Input: part model. Units: mm. Frame: model coordinates. A direction names the side the tool comes from. Coordinates: 2 decimals unless noted, no trailing zeros. Loops run counter-clockwise (first coordinate to the right, second up) from the corner with the lowest first, then second, coordinate; pieces in that order, holes last. Notation, with made-up numbers: (79.5, -3.5) -> (105.5, -3.5) arc R21 cw to (105.5, 32.5) -> close; hole circle Ø7 at (61, -17). An arc over 180 degrees is marked (long way). Put each result on its own line as item: value. Start each with the question number.
1) Set-up query: faces 1 (the flat face through (-1.5, 9, 30)), 2 (the flat face through (-33, 1.5, 8)), 3 (the flat face through (1.574, 31.563, 7.814)). Return all of +Z, -Z, +X, -X, +Y, -Y with unobstructed straight access to the full face (end or side cutting, diameter ignored); none if empty.
2) Cut plane C-C (x = -12.5). Return the cut outline in (y, z), plus the area to 3 significant figures.
3) Cut plane A-A (z = 6). Return the cut outline in (x, y), plus the area to 3 significant figures.
4) Contact query for flat-ended pins moving along their axis: P1, Ø2, axis at x = -27.5, z = 14.5, coming from the -Y side; P2, Ø8, axis at x = -32.5, y = 11, coming from the +Z side; P3, Ø2, axis at x = -19, z = 24.5, coming from the +Y side; P4, Ø13, axis at y = 11, z = 26.5, coming from the +X side. Output: stop coordinate, or through.
5) Cut plane D-D (x = -25.5). Return the cut outline in (y, z), plus the area to 3 significant figures.
6) Material intervals for L1, parallel to X at y = 15.5, z = 2; L2, parallel to Z at x = -7.5, y = 44; L3, parallel to Y at x = -3.5, z = 36, sorted ascending.
7) Cut plane B-B (y = 16). Return the cut outline in (x, z), plus the area to 3 significant figures.
from build123d import *

# Parameters (mm, degrees)
F1_DEPTH = 15.85
F3_DEPTH = 1.6
F4_W     = 16.05
F4_H     = 16.05
F5_DEPTH = 25.4


with BuildPart() as f1:
    # F0 (on Top) → F1 (new body)
    with BuildSketch(Plane.XY):
        Polygon((-19.63319, 0), (0, 0), (0, 19.05), (-1.455444, 19.412883), (4.689373, 44.058394), (-10.883874, 47.941241), (-17.02869, 23.295729), (-18.484134, 23.658612), (-19.63319, 19.05), (-19.63319, 17.55), (-45.03319, 17.55), (-45.03319, 1.5), (-19.63319, 1.5), align=None)
    extrude(amount=F1_DEPTH)

    # F2 (on face) → F3 (join)
    with BuildSketch(Plane.XY.offset(15.85)):
        Polygon((-19.63319, 1.5), (-19.63319, 0), (0, 0), (0, 19.05), (-1.455444, 19.412883), (-17.02869, 23.295729), (-18.484134, 23.658612), (-19.63319, 19.05), (-19.63319, 17.55), align=None)
    extrude(amount=F3_DEPTH)

    # F4 (on face) → F5 (join)
    with BuildSketch(Plane.XY.offset(17.45)):
        with Locations((-9.525, 9.525)):
            Rectangle(F4_W, F4_H)
    extrude(amount=F5_DEPTH)


solid = f1.part
Results found:
1. face 1: +Z, +X, +Y, -Y
1. face 2: +Z, -Z, -X, -Y
1. face 3: +Z, -Z, +X
2. outline: (0, 0) -> (41.46, 0) -> (41.46, 15.85) -> (22.17, 15.85) -> (22.17, 17.45) -> (17.55, 17.45) -> (17.55, 42.85) -> (1.5, 42.85) -> (1.5, 17.45) -> (0, 17.45) -> close
2. area: 1,100 mm2
3. outline: (-45.03, 1.5) -> (-19.63, 1.5) -> (-19.63, 0) -> (0, 0) -> (0, 19.05) -> (-1.46, 19.41) -> (4.69, 44.06) -> (-10.88, 47.94) -> (-17.03, 23.3) -> (-18.48, 23.66) -> (-19.63, 19.05) -> (-19.63, 17.55) -> (-45.03, 17.55) -> close
3. area: 1,230 mm2
4. P1: stops at y = 1.5
4. P2: stops at z = 15.85
4. P3: passes through
4. P4: stops at x = -1.5
5. outline: (1.5, 0) -> (17.55, 0) -> (17.55, 15.85) -> (1.5, 15.85) -> close
5. area: 254 mm2
6. L1: x = -45.03 to 0
6. L2: z = 0 to 15.85
6. L3: y = 1.5 to 17.55
7. outline: (-45.03, 0) -> (0, 0) -> (0, 17.45) -> (-1.5, 17.45) -> (-1.5, 42.85) -> (-17.55, 42.85) -> (-17.55, 17.45) -> (-19.63, 17.45) -> (-19.63, 15.85) -> (-45.03, 15.85) -> close
7. area: 1,150 mm2
